Autodesk Inventor part; units mm, degrees
ref_plane "YZ Plane" through (0, 0, 0) normal (1, 0, 0) x (0, 1, 0)
ref_plane "XZ Plane" through (0, 0, 0) normal (0, 1, 0) x (-1, 0, 0)
ref_plane "XY Plane" through (0, 0, 0) normal (0, 0, 1) x (1, 0, 0)
sketch "Esquisse1" plane through (0, 0, 0) normal (0, 1, 0) x (-1, 0, 0)
  line L0 (0, 0) -> (250, 0)
  line L1 (250, 0) -> (250, -32)
  line L2 (250, -32) -> (0, -32)
  line L3 (0, -32) -> (0, 0)
  circle A0 centre (2, -2) radius 1.5
  line L4 (250, -16) -> (0, -16) construction
  circle A1 centre (2, -30) radius 1.5
  circle A2 centre (51.1, -2) radius 1.5
  circle A3 centre (51.1, -30) radius 1.5
  circle A4 centre (100.2, -2) radius 1.5
  circle A5 centre (100.2, -30) radius 1.5
  circle A6 centre (149.3, -2) radius 1.5
  circle A7 centre (149.3, -30) radius 1.5
  circle A8 centre (198.4, -2) radius 1.5
  circle A9 centre (198.4, -30) radius 1.5
  circle A10 centre (247.5, -2) radius 1.5
  circle A11 centre (247.5, -30) radius 1.5
  dimension "d0" = 32
  dimension "d1" = 250
  dimension "d2" = 2
  dimension "d3" = 2
  dimension "d4" = 3
  dimension "d7" = 49.1
extrude "Extrusion1" add sketch "Esquisse1" along normal blind 1.6
sketch "Esquisse2" plane through (0, 1.6, 0) normal (0, 1, 0) x (1, 0, 0)
  circle A0 centre (-247.5, 30) radius 1.5 construction
  circle A1 centre (-247.5, 2) radius 1.5 construction
  circle A2 centre (-198.4, 30) radius 1.5 construction
  circle A3 centre (-198.4, 2) radius 1.5 construction
  circle A4 centre (-149.3, 30) radius 1.5 construction
  circle A5 centre (-149.3, 2) radius 1.5 construction
  circle A6 centre (-100.2, 30) radius 1.5 construction
  circle A7 centre (-100.2, 2) radius 1.5 construction
  circle A8 centre (-51.1, 30) radius 1.5 construction
  circle A9 centre (-51.1, 2) radius 1.5 construction
  circle A10 centre (-2, 30) radius 1.5 construction
  circle A11 centre (-2, 2) radius 1.5 construction
  line L0 (-250, 0) -> (0, 0) construction
  line L1 (0, 0) -> (0, 32) construction
  line L2 (0, 32) -> (-250, 32) construction
  line L3 (-250, 32) -> (-250, 0) construction
  line L4 (-246, 9.5) -> (-234, 9.5)
  line L5 (-234, 9.5) -> (-234, 21.5)
  line L6 (-234, 21.5) -> (-246, 21.5)
  line L7 (-246, 21.5) -> (-246, 9.5)
  dimension "d14" = 12
  dimension "d15" = 9.5
  dimension "d16" = 4
extrude "Extrusion2" add sketch "Esquisse2" along normal blind 7.7
sketch "Esquisse3" plane through (-246, 1.6, -21.5) normal (-1, 0, 0) x (0, 0, 1)
  circle A0 centre (4, 6) radius 1.1
  line L0 (-10.5, 0) -> (21.5, 0)
  line L1 (0, 0) -> (0, 7.7)
  line L2 (-10.5, -1.6) -> (21.5, -1.6)
  line L3 (5.5, -1.6) -> (5.5, 11.8569) construction
  dimension "d19" = 6
  dimension "d20" = 2.2
  dimension "d21" = 4
extrude "Extrusion3" add sketch "Esquisse3" along normal blind 7
sketch "Esquisse4" plane through (0, 1.6, 0) normal (0, 1, 0) x (1, 0, 0)
  line L0 (-246, 9.5) -> (-246, 21.5)
  line L1 (-246, 21.5) -> (-234, 21.5)
  line L2 (-234, 21.5) -> (-234, 9.5)
  line L3 (-234, 9.5) -> (-246, 9.5)
  circle A0 centre (-247.5, 30) radius 1.5
  circle A1 centre (-247.5, 2) radius 1.5
  circle A2 centre (-198.4, 30) radius 1.5
  circle A3 centre (-198.4, 2) radius 1.5
  circle A4 centre (-149.3, 30) radius 1.5
  circle A5 centre (-149.3, 2) radius 1.5
  circle A6 centre (-100.2, 30) radius 1.5
  circle A7 centre (-100.2, 2) radius 1.5
  circle A8 centre (-51.1, 30) radius 1.5
  circle A9 centre (-51.1, 2) radius 1.5
  circle A10 centre (-2, 30) radius 1.5
  circle A11 centre (-2, 2) radius 1.5
  line L4 (-250, 0) -> (0, 0)
  line L5 (0, 0) -> (0, 32)
  line L6 (0, 32) -> (-250, 32)
  line L7 (-250, 32) -> (-250, 0)
  line L8 (0, 0) -> (0, 32) construction
  line L9 (0, 16) -> (-250, 16) construction
  line L10 (-200, 19) -> (-190, 19)
  line L11 (-190, 19) -> (-190, 13)
  line L12 (-190, 13) -> (-200, 13)
  line L13 (-200, 13) -> (-200, 19)
  line L14 (-190, 16) -> (-200, 16) construction
  line L15 (-195, 19) -> (-195, 13) construction
  dimension "d24" = 10
  dimension "d26" = 6
  dimension "d29" = 55
extrude "Extrusion4" add sketch "Esquisse4" along normal blind 10 contours L10 L11 L12 L13
pattern_linear "Réseau rectangulaire1" count 7 spacing 22.1667 along (1, 0, 0) of "Extrusion4"
sketch "Esquisse6" plane through (0, 0, 0) normal (0, -1, 0) x (1, 0, 0)
  line L0 (-177.8333, -13) -> (-177.8333, -19)
  line L1 (-190, -19) -> (-190, -13)
  line L2 (-188.9167, -13) -> (-178.9167, -13)
  line L3 (-178.9167, -13) -> (-178.9167, -19)
  line L4 (-178.9167, -19) -> (-188.9167, -19)
  line L5 (-188.9167, -19) -> (-188.9167, -13)
  line L6 (-188.9167, -16) -> (-178.9167, -16) construction
  line L7 (-177.8333, -19) -> (-177.8333, -13) construction
  line L8 (-177.8333, -16) -> (-190, -16) construction
  line L9 (-190, -13) -> (-190, -19) construction
  point P0 (0, 0)
  point P1 (-183.9167, -16)
  dimension "d33" = 10
  dimension "d34" = 6
extrude "Extrusion5" add sketch "Esquisse6" along normal blind 10
sketch "Esquisse9" plane through (0, 0, 0) normal (0, -1, 0) x (1, 0, 0)
  line L0 (0, 0) -> (-250, 0)
  line L1 (-250, 0) -> (-250, -32)
  line L2 (-250, -32) -> (0, -32)
  line L3 (0, -32) -> (0, 0)
  circle A0 centre (-2, -2) radius 1.5
  circle A1 centre (-2, -30) radius 1.5
  circle A2 centre (-51.1, -2) radius 1.5
  circle A3 centre (-51.1, -30) radius 1.5
  circle A4 centre (-100.2, -30) radius 1.5
  circle A5 centre (-100.2, -2) radius 1.5
  circle A6 centre (-149.3, -2) radius 1.5
  circle A7 centre (-149.3, -30) radius 1.5
  circle A8 centre (-198.4, -2) radius 1.5
  circle A9 centre (-198.4, -30) radius 1.5
  circle A10 centre (-247.5, -2) radius 1.5
  circle A11 centre (-247.5, -30) radius 1.5
  line L4 (-178.9167, -13) -> (-178.9167, -19)
  line L5 (-178.9167, -19) -> (-188.9167, -19)
  line L6 (-188.9167, -19) -> (-188.9167, -13)
  line L7 (-188.9167, -13) -> (-178.9167, -13)
  line L8 (-178.9167, -13) -> (-178.9167, -19) construction
  line L9 (-178.9167, -16) -> (-142, -16) construction
  line L10 (-142, -1) -> (-142, -31) construction
  circle A12 centre (-173.9167, -22.5) radius 1.65
  circle A13 centre (-167.9167, -22.5) radius 1.65
  circle A14 centre (-161.9167, -22.5) radius 1.65
  circle A15 centre (-173.9167, -9.5) radius 1.65
  circle A16 centre (-167.9167, -9.5) radius 1.65
  circle A17 centre (-161.9167, -9.5) radius 1.65
  dimension "d51" = 6
  dimension "d56" = 3.3
  dimension "d57" = 13
  dimension "d58" = 5
extrude "Extrusion8" add sketch "Esquisse9" along normal blind 10 contours A12 | A13 | A14 | A15 | A16 | A17
sketch "Esquisse11" plane through (0, 1.6, 0) normal (0, 1, 0) x (1, 0, 0)
  line L0 (-57, 19) -> (-57, 13)
  line L1 (-57, 13) -> (-67, 13)
  line L2 (-67, 13) -> (-67, 19)
  line L3 (-67, 19) -> (-57, 19)
  line L4 (-79.1667, 19) -> (-79.1667, 13)
  line L5 (-79.1667, 13) -> (-89.1667, 13)
  line L6 (-89.1667, 13) -> (-89.1667, 19)
  line L7 (-89.1667, 19) -> (-79.1667, 19)
  line L8 (-101.3333, 19) -> (-101.3333, 13)
  line L9 (-101.3333, 13) -> (-111.3333, 13)
  line L10 (-111.3333, 13) -> (-111.3333, 19)
  line L11 (-111.3333, 19) -> (-101.3333, 19)
  line L12 (-123.5, 19) -> (-123.5, 13)
  line L13 (-123.5, 13) -> (-133.5, 13)
  line L14 (-133.5, 13) -> (-133.5, 19)
  line L15 (-133.5, 19) -> (-123.5, 19)
  line L16 (-145.6667, 19) -> (-145.6667, 13)
  line L17 (-145.6667, 13) -> (-155.6667, 13)
  line L18 (-155.6667, 13) -> (-155.6667, 19)
  line L19 (-155.6667, 19) -> (-145.6667, 19)
  line L20 (-167.8333, 19) -> (-167.8333, 13)
  line L21 (-167.8333, 13) -> (-177.8333, 13)
  line L22 (-177.8333, 13) -> (-177.8333, 19)
  line L23 (-177.8333, 19) -> (-167.8333, 19)
  line L24 (-190, 19) -> (-190, 13)
  line L25 (-190, 13) -> (-200, 13)
  line L26 (-200, 13) -> (-200, 19)
  line L27 (-200, 19) -> (-190, 19)
  line L28 (-246, 9.5) -> (-246, 21.5)
  line L29 (-246, 21.5) -> (-234, 21.5)
  line L30 (-234, 21.5) -> (-234, 9.5)
  line L31 (-234, 9.5) -> (-246, 9.5)
  circle A0 centre (-247.5, 30) radius 1.5
  circle A1 centre (-247.5, 2) radius 1.5
  circle A2 centre (-198.4, 30) radius 1.5
  circle A3 centre (-198.4, 2) radius 1.5
  circle A4 centre (-149.3, 30) radius 1.5
  circle A5 centre (-149.3, 2) radius 1.5
  circle A6 centre (-100.2, 30) radius 1.5
  circle A7 centre (-100.2, 2) radius 1.5
  circle A8 centre (-51.1, 30) radius 1.5
  circle A9 centre (-51.1, 2) radius 1.5
  circle A10 centre (-2, 30) radius 1.5
  circle A11 centre (-2, 2) radius 1.5
  line L32 (-250, 0) -> (0, 0)
  line L33 (0, 0) -> (0, 32)
  line L34 (0, 32) -> (-250, 32)
  line L35 (-250, 32) -> (-250, 0)
  line L36 (-52, 25) -> (0, 25)
  line L37 (0, 25) -> (0, 7)
  line L38 (0, 7) -> (-52, 7)
  line L39 (-52, 7) -> (-52, 25)
  line L40 (-52, 16) -> (0, 16) construction
  line L41 (0, 0) -> (0, 32) construction
  line L42 (0, 16) -> (-57, 16) construction
  line L43 (-57, 19) -> (-57, 13) construction
  dimension "d61" = 18
  dimension "d62" = 52
extrude "Extrusion9" add sketch "Esquisse11" along normal blind 4.5 contours L38 L39 L36 L33
sketch "Esquisse12" plane through (0, 6.1, 0) normal (0, 1, 0) x (1, 0, 0)
  line L0 (0, 25) -> (-52, 25)
  line L1 (-52, 25) -> (-52, 7)
  line L2 (-52, 7) -> (0, 7)
  line L3 (0, 7) -> (0, 25)
  line L4 (0, 32) -> (0, 0) construction
  line L5 (0, 16) -> (-52, 16) construction
  line L6 (-52, 25) -> (-52, 7) construction
  line L7 (-7.5, 12.25) -> (0, 12.25)
  line L8 (0, 12.25) -> (0, 19.75)
  line L9 (0, 19.75) -> (-7.5, 19.75)
  line L10 (-7.5, 19.75) -> (-7.5, 12.25)
  line L11 (0, 19.75) -> (1, 19.75)
  line L12 (1, 19.75) -> (1, 12.25)
  line L13 (1, 12.25) -> (0, 12.25)
  line L14 (0, 12.25) -> (0, 19.75)
  point P0 (0, 16)
  dimension "d65" = 7.5
  dimension "d66" = 7.5
  dimension "d69" = 1
extrude "Extrusion10" add sketch "Esquisse12" along normal blind 4 contours L11 L12 L13 L3 | L3 L7 L10 L9
sketch "Esquisse13" plane through (1, 6.1, -12.25) normal (1, 0, 0) x (0, 0, -1)
  line L0 (0, 0) -> (7.5, 0)
  line L1 (7.5, 0) -> (7.5, 4)
  line L2 (0, 4) -> (7.5, 4)
  line L3 (0, 0) -> (0, 4)
  line L4 (0.5, 3.5) -> (7, 3.5)
  line L5 (7, 3.5) -> (6.25, 0.5)
  line L6 (6.25, 0.5) -> (1.25, 0.5)
  line L7 (1.25, 0.5) -> (0.5, 3.5)
  line L8 (3.75, 3.5) -> (3.75, 0.5) construction
  line L9 (7.5, 4) -> (0, 4) construction
  line L10 (3.75, 4) -> (3.75, 0) construction
  line L11 (12.75, 0) -> (-5.25, 0) construction
  point P0 (-12.25, -6.1)
  dimension "d71" = 0.5
  dimension "d72" = 0.5
  dimension "d73" = 0.5
  dimension "d74" = 5
extrude "Extrusion11" cut sketch "Esquisse13" against normal blind 3 contours L4 L5 L6 L7
sketch "Esquisse14" plane through (0, 0, 0) normal (0, -1, 0) x (1, 0, 0)
  line L0 (0, -10) -> (-14, -10)
  line L1 (-14, -10) -> (-14, -22)
  line L2 (-14, -22) -> (0, -22)
  line L3 (0, -22) -> (0, -10)
  line L4 (0, -12.25) -> (0, -19.75) construction
  line L5 (0, -16) -> (-15.2374, -16) construction
  line L6 (0, -16) -> (-14, -16) construction
  line L7 (0, -32) -> (0, 0) construction
  line L8 (0.5, -22) -> (0, -22)
  line L9 (0, -22) -> (0, -10)
  line L10 (0, -10) -> (0.5, -10)
  line L11 (0.5, -10) -> (0.5, -22)
  dimension "d77" = 12
  dimension "d78" = 14
  dimension "d85" = 0.5
extrude "Extrusion12" add sketch "Esquisse14" along normal blind 6
sketch "Esquisse15" plane through (0, 0, -32) normal (1, 0, 0) x (0, 0, -1)
  line L0 (0, 0) -> (-10, 0)
  line L1 (0, 0) -> (0, 1.6)
  line L2 (-7, 1.6) -> (0, 1.6)
  line L3 (-7, 1.6) -> (-7, 6.1)
  line L4 (-12.25, 6.1) -> (-7, 6.1)
  line L5 (-19.75, 6.1) -> (-12.25, 6.1)
  line L6 (-25, 6.1) -> (-19.75, 6.1)
  line L7 (-25, 1.6) -> (-25, 6.1)
  line L8 (-32, 1.6) -> (-25, 1.6)
  line L9 (-32, 0) -> (-32, 1.6)
  line L10 (-22, -6) -> (-10, -6) construction
  line L11 (-16, -6) -> (-16, -0.2) construction
  circle A0 centre (-16, -3) radius 1.7
  line L12 (-10, 0) -> (-22, 0) construction
  line L13 (-22, 0) -> (-32, 0)
  line L14 (-10, 0) -> (-22, 0)
  dimension "d81" = 3
  dimension "d82" = 3.4
extrude "Extrusion13" cut sketch "Esquisse15" along normal mid plane 40 contours A0
sketch "Esquisse16" plane through (0, 0, 0) normal (0, -1, 0) x (1, 0, 0)
  line L0 (-142, 8) -> (-79, 8)
  line L1 (-79, 8) -> (-79, -40)
  line L2 (-79, -40) -> (-142, -40)
  line L3 (-142, -40) -> (-142, 8)
  line L4 (-79, -16) -> (-142, -16) construction
  line L5 (-250, 0) -> (-250, -32) construction
  line L6 (-250, -16) -> (0, -16) construction
  line L7 (0, -32) -> (0, -22) construction
  line L8 (-14, -10) -> (-14, -22) construction
  point P0 (0, 0)
  dimension "d86" = 63
  dimension "d87" = 48
  dimension "d91" = 108
extrude "Extrusion14" add sketch "Esquisse16" along normal blind 18
sketch "Esquisse17" plane through (0, 0, 0) normal (0, -1, 0) x (1, 0, 0)
  line L0 (-78, -26) -> (-68, -26)
  line L1 (-68, -26) -> (-68, -6)
  line L2 (-68, -6) -> (-78, -6)
  line L3 (-78, -6) -> (-78, -26)
  line L4 (-14, -22) -> (-14, -10) construction
  line L5 (-14, -16) -> (-79, -16) construction
  line L6 (-79, 0) -> (-79, -32) construction
  line L7 (-78, -16) -> (-68, -16) construction
  line L8 (0, -10) -> (0, 0) construction
  dimension "d92" = 68
  dimension "d93" = 10
  dimension "d94" = 20
extrude "Extrusion15" add sketch "Esquisse17" along normal blind 12
sketch "Esquisse18" plane through (0, 0, 0) normal (0, 1, 0) x (1, 0, 0)
  line L0 (-142, 32) -> (-79, 32)
  line L1 (-79, 32) -> (-79, 40)
  line L2 (-79, 40) -> (-142, 40)
  line L3 (-142, 40) -> (-142, 32)
  line L4 (-79, 0) -> (-142, 0)
  line L5 (-142, 0) -> (-142, -8)
  line L6 (-142, -8) -> (-79, -8)
  line L7 (-79, -8) -> (-79, 0)
  point P0 (0, 0)
extrude "Extrusion16" cut sketch "Esquisse18" against normal blind 3
equation "\"d72\" = d71"
equation "\"d73\" = d71"
properties part number "electronics"
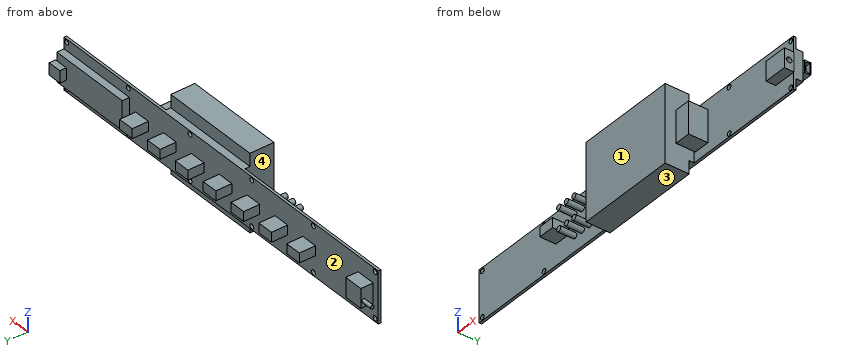
Part model, mm, in its own coordinate system. Face numbers are marked on the shaded views. A direction names the side the tool comes from. Coordinates: 2 decimals unless noted, no trailing zeros. Write each loop counter-clockwise with the first axis right and the second up, starting at its lowest first coordinate (ties: lowest second). Pieces come first, ordered by that corner, then holes.
Item 1: Slice it at B-B (x = -92). Write the cut outline in (y, z).
Item 2: Probe line 1 (Z direction, x = -100.2, y = 1.05); line 2 (Y direction, x = -28, z = -30.5); line 3 (X direction, y = -1.5, z = -25.5). List the from-to ranges inside material, lowest first.
Item 3: Slice it at C-C (x = -216). Write the cut outline in (y, z), and give its area (3 significant figures).
Item 4: Slice it at A-A (x = -23). Write the cut outline in (y, z), and give its area (3 significant figures).
Item 5: Pin check, flat tips, straight feed: pin 1 (8 mm diameter, centred on x = -27, z = -10, fed in from +Y); pin 2 (1.6 mm diameter, centred on x = -173.5, z = -22.5, fed in from -Y); pin 3 (5 mm diameter, centred on x = -22, y = 4, fed in from +Z). Stop position of each tip, or through.
Item 6: Mould opens along X. For the marked faces 1 and 2 say: released by +X, released by -X, zero draft, split by the parting line, or undercut.
Item 7: Which spindle directions (+Z, -Z, +X, -X, +Y, -Y) get a long thin tool onto all of the face, cutting with end or side? Do the marked faces 3 and 4. Say none if no direction does.
Results found:
1. outline: (-18, -40) - (-3, -40) - (-3, -32) - (1.6, -32) - (1.6, 0) - (-3, 0) - (-3, 8) - (-18, 8) - close
2. line 1: z = -32 to -31.5, -28.5 to -3.5, -0.5 to 0
2. line 2: y = 0 to 1.6
2. line 3: x = -142 to -79, -78 to -68
3. outline: (0, -32) - (1.6, -32) - (1.6, 0) - (0, 0) - close
3. area: 51.2 mm2
4. outline: (0, -32) - (1.6, -32) - (1.6, -25) - (6.1, -25) - (6.1, -7) - (1.6, -7) - (1.6, 0) - (0, 0) - close
4. area: 132 mm2
5. pin 1: stops at y = 6.1
5. pin 2: stops at y = -10
5. pin 3: stops at z = 0
6. face 1: zero draft
6. face 2: undercut
7. face 3: -Z, +X, -X, +Y, -Y
7. face 4: +Z, -Z, -Y
